The drawing under review shows one solid part. Ordinate dimensions are in mm from its lowest x, y, z. A direction names the side the tool comes from. Give positions to 0.01 mm unless a question says otherwise; leave off trailing zeros. Loops run counter-clockwise (first coordinate to the right, second up) from the corner with the lowest first, then second, coordinate; pieces in that order, holes last. Notation, with made-up numbers: (11, -18) - (66, -18) arc R21 ccw to (66, 1) - close; hole circle Ø11 at (-4.75, -36). An arc over 180 degrees is marked (long way). Return JSON: item names as keys, results as strings. Group by question number.
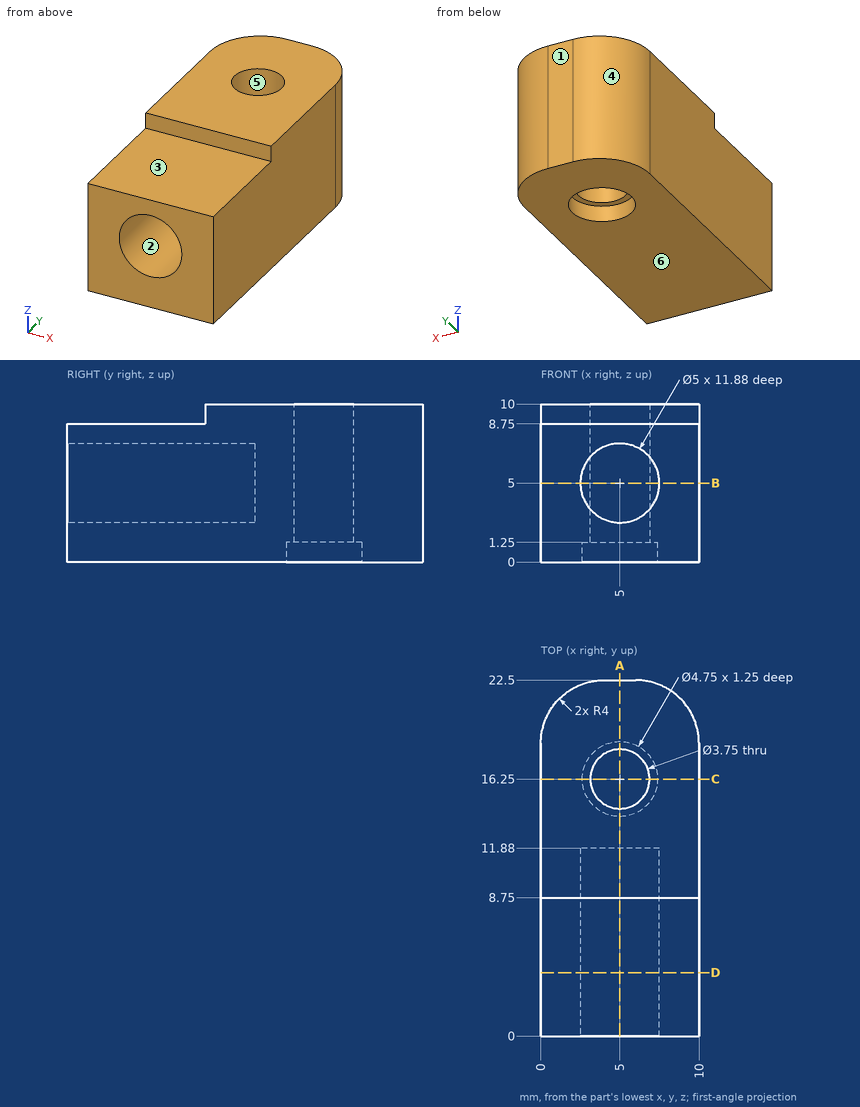
1) We need section C-C, the plane y = 16.25. Write out the cut boundary in (x, z) (3 decimals), plus the area to 4 significant figures.
2) For pin 1 Ø5 at (x, y) = (1.5, 9) entering from -Z; pin 2 Ø1.4 at (x, z) = (5.5, 9.5) entering from -Y; pin 3 Ø2 at (x, y) = (5, 16.25) entering from +Z; pin 4 Ø1.5 at (x, z) = (5.5, 4.5) entering from -Y, all flat-tipped, find the tip position at first contact; note any pin that passes through.
3) To check wall thickness, follow line 1 (Y direction, x = 5, z = 6.25) (3 decimals); line 2 (Y direction, x = 5, z = 0.55) (3 decimals); line 3 (Z direction, x = 5, y = 5). State the ranges of each line that lie inside material, in increasing order.
4) We need section A-A, the plane x = 5. Write out the cut boundary in (y, z) (3 decimals), plus the area to 3 significant figures.
5) We need section B-B, the plane z = 5. Write out the cut boundary in (x, y) (3 decimals), plus the area to 3 significant figures.
6) We need section D-D, the plane y = 4. Write out the cut boundary in (x, z).
7) Draft analysis for pull direction X (two halves, no side actions). For the marked faces 4, 5 and 6, state which applies: +X half, -X half, draft (parallel to the pull), parting line (faces both ways), or undercut.
8) Tool access review of the marked faces 1, 2 and 3: name each direction out of +Z, -Z, +X, -X, +Y, -Y from which nothing blocks a thin tool from reaching the whole face with its end or side.
Findings:
{
 "1": {"outline": "(0, 0) - (2.625, 0) - (2.625, 1.25) - (3.125, 1.25) - (3.125, 10) - (0, 10) - close; (6.875, 1.25) - (7.375, 1.25) - (7.375, 0) - (10, 0) - (10, 10) - (6.875, 10) - close", "area": "61.25 mm^2"},
 "2": {"pin 1": "stops at z = 0", "pin 2": "stops at y = 8.75", "pin 3": "passes through", "pin 4": "stops at y = 11.88"},
 "3": {"line 1": "y = 11.88 to 14.375, 18.125 to 22.5", "line 2": "y = 0 to 13.875, 18.625 to 22.5", "line 3": "z = 0 to 2.5, 7.5 to 8.75"},
 "4": {"outline": "(0, 0) - (13.875, 0) - (13.875, 1.25) - (14.375, 1.25) - (14.375, 10) - (8.75, 10) - (8.75, 8.75) - (0, 8.75) - (0, 7.5) - (11.88, 7.5) - (11.88, 2.5) - (0, 2.5) - close; (18.125, 1.25) - (18.625, 1.25) - (18.625, 0) - (22.5, 0) - (22.5, 10) - (18.125, 10) - close", "area": "116 mm^2"},
 "5": {"outline": "(0, 0) - (2.5, 0) - (2.5, 11.88) - (7.5, 11.88) - (7.5, 0) - (10, 0) - (10, 18.5) arc R4 ccw to (6, 22.5) - (4, 22.5) arc R4 ccw to (0, 18.5) - close; hole circle Ø3.75 at (5, 16.25)", "area": "148 mm^2"},
 "6": {"outline": "(0, 0) - (10, 0) - (10, 8.75) - (0, 8.75) - close; hole circle Ø5 at (5, 5)"},
 "7": {"face 4": "-X half", "face 5": "undercut", "face 6": "draft"},
 "8": {"face 1": "+Z, -Z, +X, -X, +Y", "face 2": "-Y", "face 3": "+Z, +X, -X, -Y"}
}
